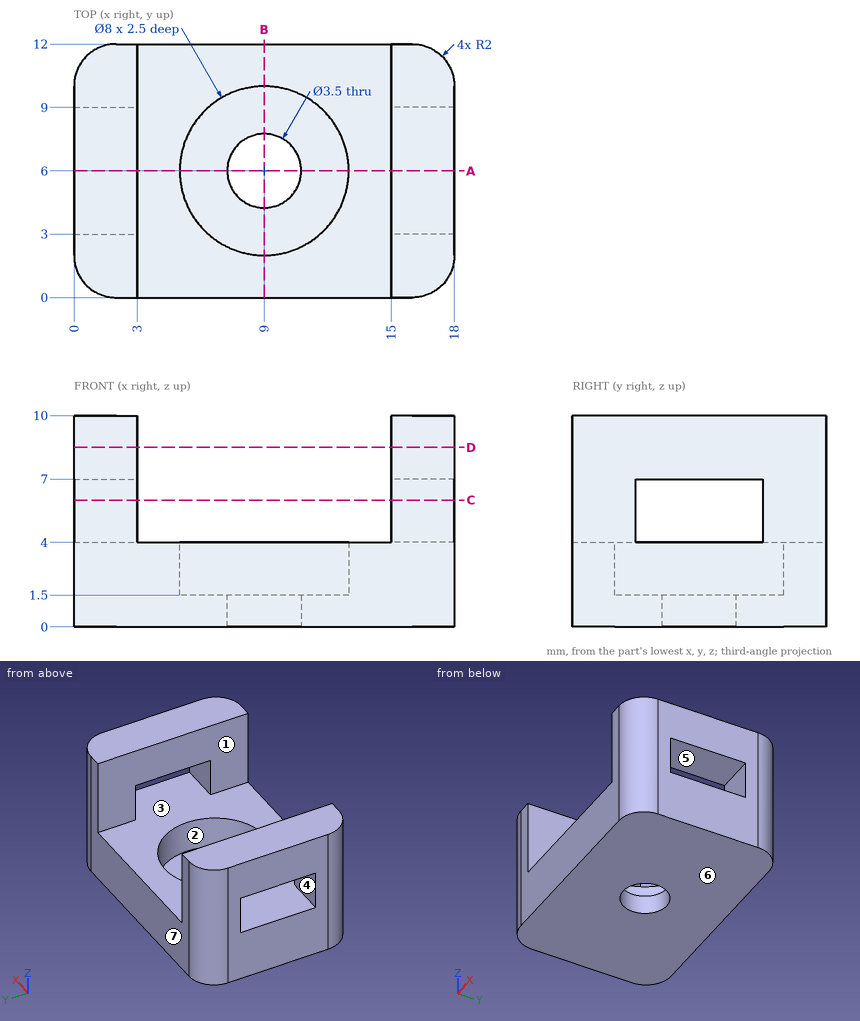
For this review, use the dimensioned drawing (mm, ordinates from the lowest corner) and the shaded views. A direction names the side the tool comes from. Round coordinates to 2 decimals unless told otherwise and drop trailing zeros. Write each loop counter-clockwise with the first axis right and the second up, starting at its lowest first coordinate (ties: lowest second). Pieces come first, ordered by that corner, then holes. Notation, with made-up numbers: (26.25, -17.75) - (81.25, -17.75) arc R10 cw to (81.25, -9.75) - close; hole circle Ø7 at (12, 36.25). An arc over 180 degrees is marked (long way). Use a Markdown table: item, result.
Q1. Clearance check with a flat-ended pin moving along its axis: pin 1 (7 mm diameter, centred on x = 9, y = 6, fed in from +Z). State where the tip first meets the part, or that it passes through.
Derived:
| item | result |
|---|---|
| pin 1 | stops at z = 1.5 |
Q2. We need section B-B (x = 9). Give the boundary of the cut face in (y, z).
Derived:
| item | result |
|---|---|
| outline | (0, 0) - (4.25, 0) - (4.25, 1.5) - (2, 1.5) - (2, 4) - (0, 4) - close; (7.75, 0) - (12, 0) - (12, 4) - (10, 4) - (10, 1.5) - (7.75, 1.5) - close |
Q3. The part is to be moulded in two halves that separate along Z. For the marked faces 5, 6 and 7, say which applies: pulls with the +Z half, pulls with the -Z half, needs draft (parallel to the pull), parting line crosses it, or undercut.
Derived:
| item | result |
|---|---|
| face 5 | undercut |
| face 6 | pulls with the -Z half |
| face 7 | needs draft |
Q4. We need section A-A (y = 6). Give the boundary of the cut face in (x, z), plus the area to 4 significant figures.
Derived:
| item | result |
|---|---|
| outline | (0, 0) - (7.25, 0) - (7.25, 1.5) - (5, 1.5) - (5, 4) - (0, 4) - close; (0, 7) - (3, 7) - (3, 10) - (0, 10) - close; (10.75, 0) - (18, 0) - (18, 4) - (13, 4) - (13, 1.5) - (10.75, 1.5) - close; (15, 7) - (18, 7) - (18, 10) - (15, 10) - close |
| area | 64.75 mm2 |
Q5. We need section C-C (z = 6). Give the boundary of the cut face in (x, y).
Derived:
| item | result |
|---|---|
| outline | (0, 2) arc R2 ccw to (2, 0) - (3, 0) - (3, 3) - (0, 3) - close; (0, 9) - (3, 9) - (3, 12) - (2, 12) arc R2 ccw to (0, 10) - close; (15, 0) - (16, 0) arc R2 ccw to (18, 2) - (18, 3) - (15, 3) - close; (15, 9) - (18, 9) - (18, 10) arc R2 ccw to (16, 12) - (15, 12) - close |
Q6. Wall thickness on line 1 along X through (y, z) = (7.5, 8.25); line 2 along Y through (x, z) = (9, 0.65); line 3 along Y through (x, z) = (9, 2.5): over which ranges is each line inside the solid? List them lowest first.
Derived:
| item | result |
|---|---|
| line 1 | x = 0 to 3, 15 to 18 |
| line 2 | y = 0 to 4.25, 7.75 to 12 |
| line 3 | y = 0 to 2, 10 to 12 |
Q7. We need section D-D (z = 8.5). Give the boundary of the cut face in (x, y).
Derived:
| item | result |
|---|---|
| outline | (0, 2) arc R2 ccw to (2, 0) - (3, 0) - (3, 12) - (2, 12) arc R2 ccw to (0, 10) - close; (15, 0) - (16, 0) arc R2 ccw to (18, 2) - (18, 10) arc R2 ccw to (16, 12) - (15, 12) - close |
Q8. Machinability: for the marked faces 1, 2, 3 and 4, which of the approach directions +Z, -Z, +X, -X, +Y, -Y give a long, thin tool a straight path to every point of the face, cutting with its end or side? Answer none if there is none.
Derived:
| item | result |
|---|---|
| face 1 | +Z, +Y, -Y |
| face 2 | +Z |
| face 3 | none |
| face 4 | +X, -X |
